Check sheet for the drawn part. Datum: minimum x, y, z corner. Units: mm. A direction names the side the tool comes from. Give positions to 0.01 mm unless a question says otherwise; leave off trailing zeros. Loops run counter-clockwise (first coordinate to the right, second up) from the corner with the lowest first, then second, coordinate; pieces in that order, holes last. Notation, with made-up numbers: (2, -11.5) - (56, -11.5) arc R17 cw to (56, 0.5) - close; hole circle Ø1 at (87.5, -4). An arc over 180 degrees is marked (long way). Use one line per item in the form item = value.
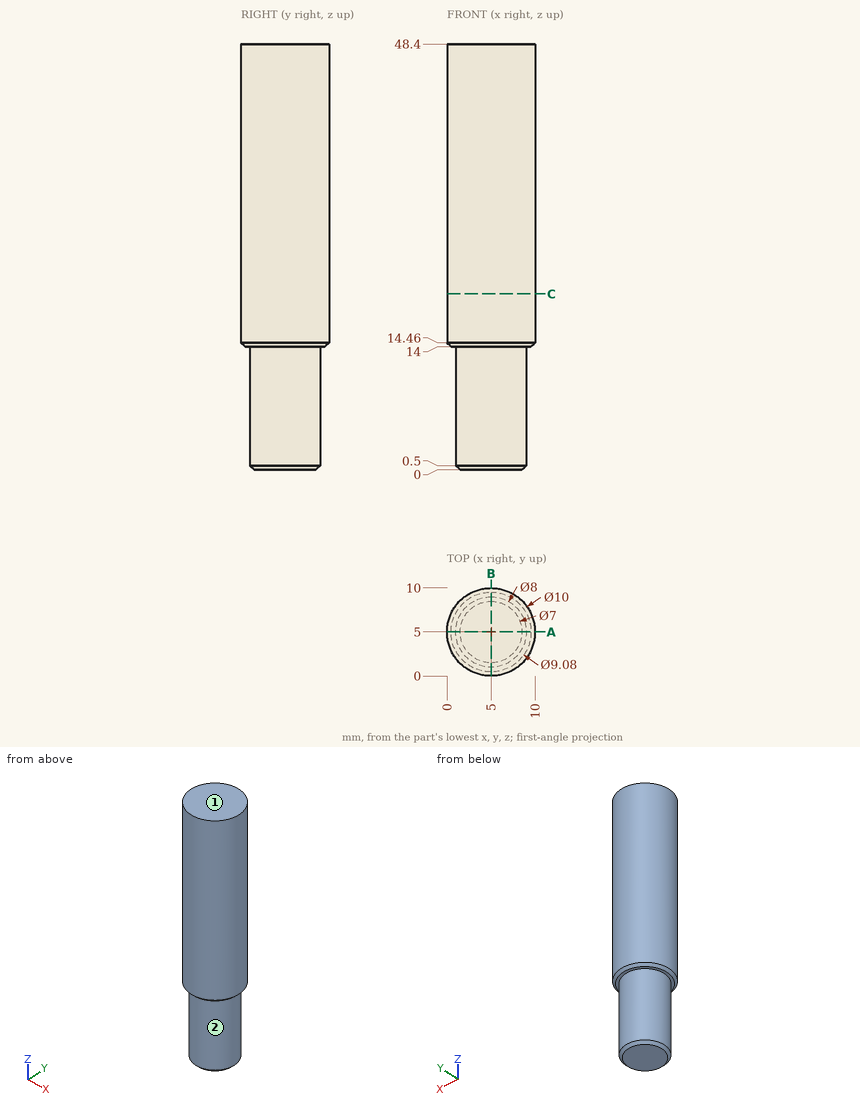
1. Section check A-A, the plane y = 5. Record the cut outline in (x, z).
Result set:
outline = (0, 14.46) - (0.46, 14) - (1, 14) - (1, 0.5) - (1.5, 0) - (8.5, 0) - (9, 0.5) - (9, 14) - (9.54, 14) - (10, 14.46) - (10, 48.4) - (0, 48.4) - close
2. Tool access check on the marked faces 1 and 2. Record the directions out of +Z, -Z, +X, -X, +Y, -Y that give a thin tool (end or side, any length) a straight path to the whole face; none if there is none.
Result set:
face_1 = +Z, +X, -X, +Y, -Y
face_2 = -Z
3. Section check C-C, the plane z = 20. Record the cut outline in (x, y).
Result set:
outline = circle Ø10 at (5, 5)
4. Depth check by flat-ended pin: pin 1 Ø4 at (x, z) = (7.5, 39.5) entering from -Y; pin 2 Ø1.5 at (x, y) = (1.5, 2) entering from -Z; pin 3 Ø4 at (y, z) = (1, 36.5) entering from -X. Enter the tip coordinate at first touch or a pass-through.
Result set:
pin_1 = 0.03
pin_2 = 0.36
pin_3 = 0.42
5. Scan lines: probe 1 along X at (y, z) = (7, 24); probe 2 along Y at (x, z) = (4.5, 31); probe 3 along Y at (x, z) = (9.5, 35.5). Record each from-to range of solid material in increasing order.
Result set:
probe_1 = 0.42 to 9.58
probe_2 = 0.03 to 9.97
probe_3 = 2.82 to 7.18
